Part print with two shaded views. Sizes in mm from the minimum x, y, z corner. A direction names the side the tool comes from. Round coordinates to 2 decimals unless told otherwise and drop trailing zeros. Loops run counter-clockwise (first coordinate to the right, second up) from the corner with the lowest first, then second, coordinate; pieces in that order, holes last.
(1) Cut at D-D on z = 26. List the corners of the cut face in (x, y), then the cut area to 3 significant figures.
(2) Cut at C-C on x = 26.5. List the corners of the cut face in (y, z).
(3) Cut at A-A on z = 6. List the corners of the cut face in (x, y).
(4) Cut at B-B on y = 7. List the corners of the cut face in (x, z).
(5) Probe probe 1 along Z at (x, y) = (1, 7); probe 2 along X at (y, z) = (13.25, 8.75); probe 3 along Z at (x, y) = (38, 12.5). List the from-to ranges inside material, lowest first.
(6) Flat gauge pins, fed straight in: pin 1 (12 mm diameter, centred on x = 26, y = 8, fed in from +Z); pin 2 (0.6 mm diameter, centred on x = 52, z = 18.5, fed in from +Y); pin 3 (1.9 mm diameter, centred on y = 7, z = 23, fed in from +X); pin 4 (13 mm diameter, centred on x = 35.5, y = 18.5, fed in from +Z). Where does each tip first touch, or does it go through?
(7) Mould opens along X. For the marked faces 4, 5 and 6 say: +X half, -X half, draft (parallel to the pull), parting line (faces both ways), or undercut.
(8) Tool access for the marked faces 1, 2 and 3: list every direction of +Z, -Z, +X, -X, +Y, -Y with a clear straight run to the whole face (end or side of a thin tool).
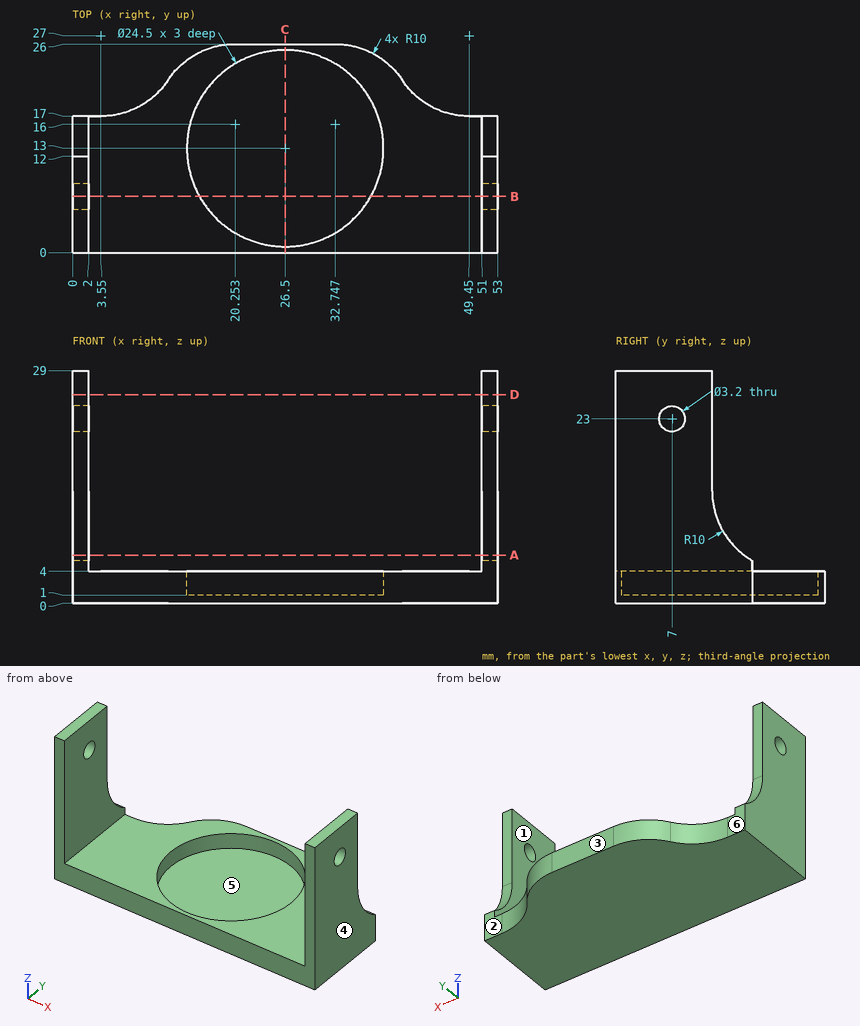
Final values:
1. outline: (0, 0) - (2, 0) - (2, 12) - (0, 12) - close; (51, 0) - (53, 0) - (53, 12) - (51, 12) - close
1. area: 48.0 mm2
2. outline: (0, 0) - (26, 0) - (26, 4) - (25.25, 4) - (25.25, 1) - (0.75, 1) - (0.75, 4) - (0, 4) - close
3. outline: (0, 0) - (2, 0) - (2, 16) - (0, 16) - close; (51, 0) - (53, 0) - (53, 16) - (51, 16) - close
4. outline: (0, 0) - (53, 0) - (53, 21.4) - (51, 21.4) - (51, 4) - (37.18, 4) - (37.18, 1) - (15.82, 1) - (15.82, 4) - (2, 4) - (2, 21.4) - (0, 21.4) - close; (0, 24.6) - (2, 24.6) - (2, 29) - (0, 29) - close; (51, 24.6) - (53, 24.6) - (53, 29) - (51, 29) - close
5. probe 1: z = 0 to 21.4, 24.6 to 29
5. probe 2: x = 0 to 2, 51 to 53
5. probe 3: z = 0 to 1
6. pin 1: stops at z = 1
6. pin 2: stops at y = 12
6. pin 3: passes through
6. pin 4: stops at z = 4
7. face 4: +X half
7. face 5: undercut
7. face 6: draft
8. face 1: +Z, +Y, -Y
8. face 2: +Z, -Z, +X, +Y
8. face 3: +Z, -Z, +X, -X, +Y
